Could you check a few things on this model? Use its own coordinates, in mm. Face numbers are marked on the shaded views. A direction names the side the tool comes from. Give positions to 0.01 mm unless a question says otherwise; leave off trailing zeros. Order: outer loops, then holes, each group sorted by start corner. A loop starts at its lowest first (then second) coordinate and runs counter-clockwise, first axis right, second up. Notation, with made-up numbers: (9, 75.25) -> (57, 75.25) arc R15 cw to (57, 99.25) -> close; hole circle Ø10 at (15, -8.5). An arc over 180 degrees is marked (long way). Write each question's results on one line, items separated by ' | '.
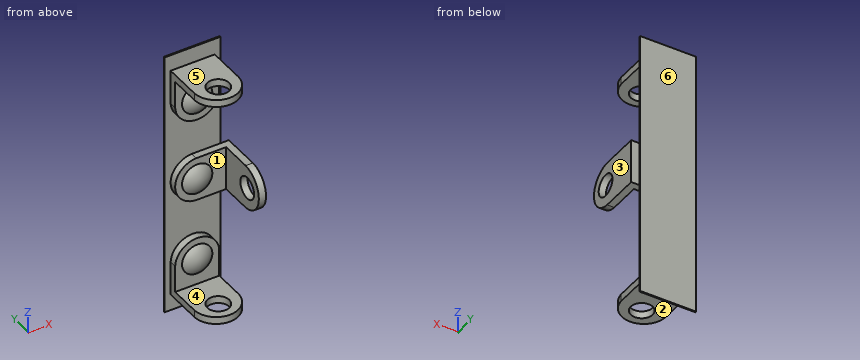
```python
from build123d import *

# Parameters (mm, degrees)
SKETCH1_W           = 6.096
SKETCH1_H           = 29.21
BOSS_EXTRUDE1_DEPTH = 0.127
BOSS_EXTRUDE2_DEPTH = 0.7874
BOSS_EXTRUDE3_DEPTH = 0.7874
BOSS_EXTRUDE4_DEPTH = 0.7874
SKETCH5_R           = 1.1938
BOSS_EXTRUDE5_DEPTH = 0.7874
SKETCH6_R           = 1.1938
BOSS_EXTRUDE6_DEPTH = 0.7874
SKETCH7_R           = 1.1938
BOSS_EXTRUDE7_DEPTH = 0.7874


with BuildPart() as part:
    # Sketch1 → Boss-Extrude1 (new body)
    with BuildSketch(Plane(origin=(0, 0, 0), x_dir=(1, 0, 0), z_dir=(0, 1, 0))):
        Rectangle(SKETCH1_W, SKETCH1_H)
    extrude(amount=BOSS_EXTRUDE1_DEPTH)

    # Sketch2 → Boss-Extrude2 (add)
    with BuildSketch(Plane(origin=(0, 0, 0), x_dir=(1, 0, 0), z_dir=(0, 1, 0))):
        with BuildLine():
            Line((-0.1171575, -2.4003), (3.5404425, -2.4003))
            Line((3.5404425, -2.4003), (3.5404425, 2.4003))
            Line((3.5404425, 2.4003), (-0.1171575, 2.4003))
            ThreePointArc((-0.1171575, 2.4003), (-2.4031575, 0), (-0.1171575, -2.4003))
        make_face()
    extrude(amount=-BOSS_EXTRUDE2_DEPTH)

    # Sketch3 → Boss-Extrude3 (add)
    with BuildSketch(Plane(origin=(0, 0, 0), x_dir=(1, 0, 0), z_dir=(0, 1, 0))):
        with BuildLine():
            Line((2.4003, 9.0776425), (2.4003, 12.7352425))
            Line((2.4003, 12.7352425), (-2.4003, 12.7352425))
            Line((-2.4003, 12.7352425), (-2.4003, 9.0776425))
            ThreePointArc((-2.4003, 9.0776425), (0, 6.7916425), (2.4003, 9.0776425))
        make_face()
    extrude(amount=-BOSS_EXTRUDE3_DEPTH)

    # Sketch4 → Boss-Extrude4 (add)
    with BuildSketch(Plane(origin=(0, 0, 0), x_dir=(1, 0, 0), z_dir=(0, 1, 0))):
        with BuildLine():
            Line((-2.4003, -12.7352425), (2.4003, -12.7352425))
            Line((2.4003, -12.7352425), (2.4003, -9.0776425))
            ThreePointArc((2.4003, -9.0776425), (0, -6.7916425), (-2.4003, -9.0776425))
            Line((-2.4003, -9.0776425), (-2.4003, -12.7352425))
        make_face()
    extrude(amount=-BOSS_EXTRUDE4_DEPTH)

    # Sketch5 → Boss-Extrude5 (add)
    with BuildSketch(Plane(origin=(3.937, 0, 0), x_dir=(0, 0, -1), z_dir=(1, 0, 0))):
        with BuildLine():
            Line((-2.4003, 0), (-2.4003, -4.191))
            ThreePointArc((-2.4003, -4.191), (0, -6.477), (2.4003, -4.191))
            Line((2.4003, -4.191), (2.4003, 0))
            Line((2.4003, 0), (-2.4003, 0))
        make_face()
        with Locations((0, -4.4577)):
            Circle(SKETCH5_R, mode=Mode.SUBTRACT)
    extrude(amount=-BOSS_EXTRUDE5_DEPTH)

    # Sketch6 → Boss-Extrude6 (add)
    with BuildSketch(Plane.XY.offset(12.827)):
        with BuildLine():
            Line((-2.4003, 0), (-2.4003, -4.191))
            ThreePointArc((-2.4003, -4.191), (0, -6.477), (2.4003, -4.191))
            Line((2.4003, -4.191), (2.4003, 0))
            Line((2.4003, 0), (-2.4003, 0))
        make_face()
        with Locations((0, -4.4577)):
            Circle(SKETCH6_R, mode=Mode.SUBTRACT)
    extrude(amount=-BOSS_EXTRUDE6_DEPTH)

    # Sketch7 → Boss-Extrude7 (add)
    with BuildSketch(Plane.XY.offset(-12.827)):
        with BuildLine():
            Line((-2.4003, 0), (-2.4003, -4.191))
            ThreePointArc((-2.4003, -4.191), (0, -6.477), (2.4003, -4.191))
            Line((2.4003, -4.191), (2.4003, 0))
            Line((2.4003, 0), (-2.4003, 0))
        make_face()
        with Locations((0, -4.4577)):
            Circle(SKETCH7_R, mode=Mode.SUBTRACT)
    extrude(amount=BOSS_EXTRUDE7_DEPTH)

    # Sketch8 → Revolve1 (revolve)
    with BuildSketch(Plane.XY):
        with BuildLine():
            Line((0, 0), (1.651, 0))
            Line((1.651, 0), (1.651, -0.7874))
            ThreePointArc((1.651, -0.7874), (0.871501354, -1.202713091), (0, -1.3462))
            Line((0, -1.3462), (0, 0))
        make_face()
    revolve(axis=Axis((0, -1.3462, 0), (0, 1, 0)))

    # Sketch9 → Revolve2 (revolve)
    with BuildSketch(Plane(origin=(0, 0, 0), x_dir=(0, 0, -1), z_dir=(1, 0, 0))):
        with BuildLine():
            Line((9.1948, 0), (10.8458, 0))
            Line((10.8458, 0), (10.8458, -0.7874))
            ThreePointArc((10.8458, -0.7874), (10.066301354, -1.202713091), (9.1948, -1.3462))
            Line((9.1948, -1.3462), (9.1948, 0))
        make_face()
    revolve(axis=Axis((0, -1.3462, -9.1948), (0, 1, 0)))

    # Sketch10 → Revolve3 (revolve)
    with BuildSketch(Plane(origin=(0, 0, 0), x_dir=(0, 0, -1), z_dir=(1, 0, 0))):
        with BuildLine():
            Line((-9.1948, 0), (-7.5438, 0))
            Line((-7.5438, 0), (-7.5438, -0.7874))
            ThreePointArc((-7.5438, -0.7874), (-8.323298646, -1.202713091), (-9.1948, -1.3462))
            Line((-9.1948, -1.3462), (-9.1948, 0))
        make_face()
    revolve(axis=Axis((0, -1.3462, 9.1948), (0, 1, 0)))


solid = part.part
```
Q1. I need wall thicknesses on line 1 along Z through (x, y) = (-1, -3.25); line 2 along Y through (x, z) = (3.8, 0); line 3 along Z through (x, y) = (3.75, -4.25). Which ranges of each line are inside material? Lowest first, please.
Here are the results:
line 1: z = -12.83 to -12.04, 12.04 to 12.83 | line 2: y = -6.48 to -5.65, -3.26 to 0 | line 3: z = -2.4 to -1.18, 1.18 to 2.4
Q2. Suppose I cut it at A-A on y = -2.25. Please give me the cut outline in (x, z), and give its area (3 significant figures).
Here are the results:
outline: (-2.4, -12.83) -> (2.4, -12.83) -> (2.4, -12.04) -> (-2.4, -12.04) -> close; (-2.4, 12.04) -> (2.4, 12.04) -> (2.4, 12.83) -> (-2.4, 12.83) -> close; (3.15, -2.4) -> (3.94, -2.4) -> (3.94, 2.4) -> (3.15, 2.4) -> close | area: 11.3 mm²
Q3. Suppose I cut it at B-B on z = 0. Please give me the cut outline in (x, y).
Here are the results:
outline: (-3.05, 0) -> (-2.4, 0) -> (-2.4, -0.79) -> (-1.65, -0.79) arc R2.72 ccw to (1.65, -0.79) -> (3.15, -0.79) -> (3.15, -3.26) -> (3.94, -3.26) -> (3.94, 0) -> (3.05, 0) -> (3.05, 0.13) -> (-3.05, 0.13) -> close; (3.15, -6.48) -> (3.94, -6.48) -> (3.94, -5.65) -> (3.15, -5.65) -> close
Q4. For the marked faces 5 and 6, which set-ups out of +Z, -Z, +X, -X, +Y, -Y let a thin tool reach every point of the face, with its end or its side?
Here are the results:
face 5: +Z, +X, -X, -Y | face 6: +Z, -Z, +X, -X, +Y
Q5. Suppose I cut it at C-C on x = -0.75. State how many separate pieces and enclosed holes the cut face has, and give its area (3 significant figures).
Here are the results:
separate pieces: 3 | enclosed holes: 0 | area: 25.2 mm²
Q6. Thinking about a two-plate mould opening in Z: for the marked faces 1, 2, 3 and 4, which applies, +Z half, -Z half, draft (parallel to the pull), parting line (faces both ways), or undercut?
Here are the results:
face 1: undercut | face 2: -Z half | face 3: draft | face 4: undercut
Q7. I'm going to push flat-ended pins straight in: pin 1 Ø0.7 at (x, z) = (3.5, 1) entering from +Y; pin 2 Ø4 at (x, z) = (0, -1) entering from -Y; pin 3 Ø1 at (x, z) = (0, 4) entering from -Y; pin 4 Ø1.1 at (y, z) = (-2, -10.5) entering from -X. Where does each tip first touch, or does it pass through?
Here are the results:
pin 1: stops at y = 0 | pin 2: stops at y = -1.35 | pin 3: stops at y = 0 | pin 4: passes through
Q8. Suppose I cut it at D-D on x = -2. Please give me the cut outline in (y, z) (3 decimals), and give its area (3 significant figures).
Here are the results:
outline: (-5.406, -12.827) -> (0, -12.827) -> (0, -14.605) -> (0.127, -14.605) -> (0.127, 14.605) -> (0, 14.605) -> (0, 12.827) -> (-5.406, 12.827) -> (-5.406, 12.04) -> (-0.787, 12.04) -> (-0.787, 7.862) -> (0, 7.862) -> (0, 1.332) -> (-0.787, 1.332) -> (-0.787, -1.332) -> (0, -1.332) -> (0, -7.862) -> (-0.787, -7.862) -> (-0.787, -12.04) -> (-5.406, -12.04) -> close | area: 20.9 mm²
